Could you check a few things on this drawing? It's one solid part, dimensions in mm from its lowest x, y, z. A direction names the side the tool comes from. Coordinates: 2 decimals unless noted, no trailing zeros. Loops run counter-clockwise (first coordinate to the right, second up) from the corner with the lowest first, then second, coordinate; pieces in that order, holes last.
1) Imagine slicing it at C-C on z = 3. Please give me the cut outline in (x, y), plus the area to 3 significant figures.
2) Imagine slicing it at A-A on y = 10.75. Please give me the cut outline in (x, z).
3) If I drill on line 1 along Z through (x, y) = (15, 14.5); line 2 along Z through (x, y) = (14.5, 17.75); line 3 along Y through (x, z) = (9.5, 1.5), over which ranges is the centre line in solid material (lowest first)?
4) Will these pins go through, and if not, where does the flat tip stop? P1, Ø2, axis at x = 4.5, z = 0.5, coming from the +Y side; P2, Ø12, axis at x = 3, y = 8.5, coming from the +Z side; P3, Ø1.5, axis at x = 7, z = 3.5, coming from the -Y side; P4, Ø2, axis at x = 5, z = 2.5, coming from the +Y side.
5) For the marked faces 1 and 2, which set-ups out of +Z, -Z, +X, -X, +Y, -Y let a thin tool reach every point of the face, with its end or its side?
6) Imagine slicing it at D-D on y = 5. Please give me the cut outline in (x, z), plus the area to 3 significant figures.
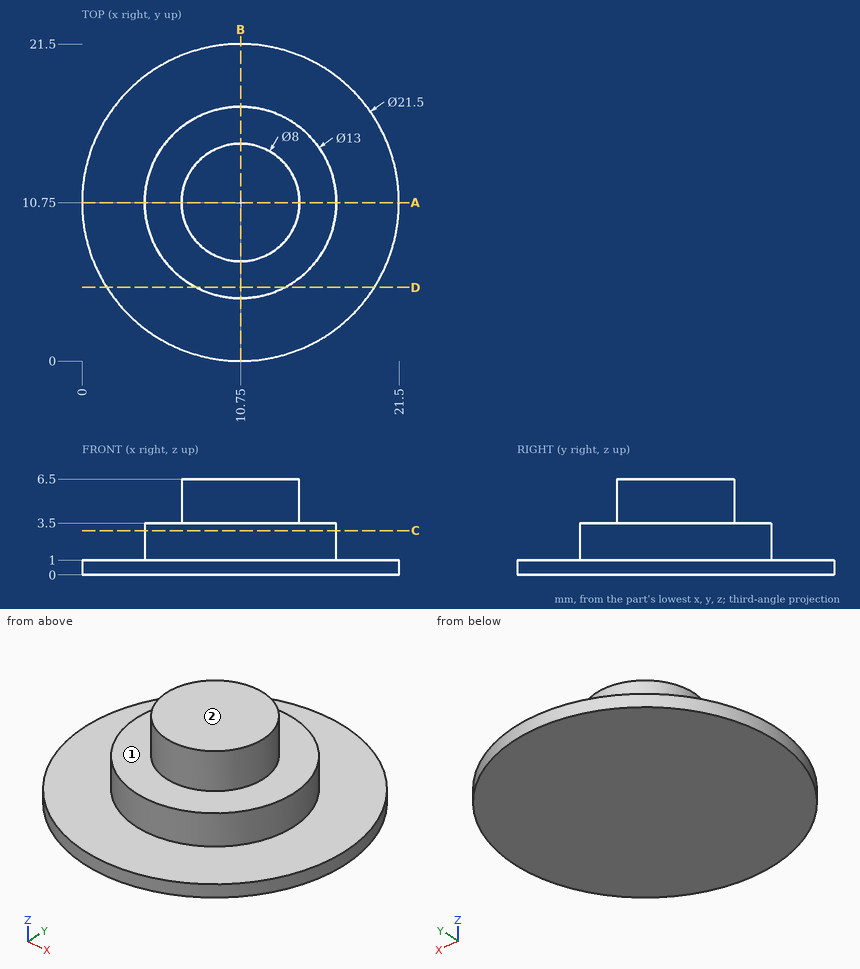
Filled in:
1. outline: circle Ø13 at (10.75, 10.75)
1. area: 133 mm2
2. outline: (0, 0) - (21.5, 0) - (21.5, 1) - (17.25, 1) - (17.25, 3.5) - (14.75, 3.5) - (14.75, 6.5) - (6.75, 6.5) - (6.75, 3.5) - (4.25, 3.5) - (4.25, 1) - (0, 1) - close
3. line 1: z = 0 to 3.5
3. line 2: z = 0 to 1
3. line 3: y = 4.37 to 17.13
4. P1: stops at y = 20.13
4. P2: stops at z = 6.5
4. P3: stops at y = 4.98
4. P4: stops at y = 15.19
5. face 1: +Z
5. face 2: +Z, +X, -X, +Y, -Y
6. outline: (1.67, 0) - (19.83, 0) - (19.83, 1) - (13.78, 1) - (13.78, 3.5) - (7.72, 3.5) - (7.72, 1) - (1.67, 1) - close
6. area: 33.3 mm2
